```python
from build123d import *

# Parameters (mm, degrees)
SKETCH_1_W      = 60
SKETCH_1_H      = 60
EXTRUDE_1_DEPTH = 3
SKETCH_2_W      = 60
SKETCH_2_H      = 60
EXTRUDE_2_DEPTH = 35
EXTRUDE_3_DEPTH = 8


with BuildPart() as part:
    # 草图1 → 凸台-拉伸1 (new body)
    with BuildSketch(Plane(origin=(0, 0, 0), x_dir=(1, 0, 0), z_dir=(0, 1, 0))):
        Rectangle(SKETCH_1_W, SKETCH_1_H)
    extrude(amount=EXTRUDE_1_DEPTH)

    # 草图2 → 凸台-拉伸2 (add)
    with BuildSketch(Plane(origin=(0, 0, 0), x_dir=(1, 0, 0), z_dir=(0, 1, 0))):
        Polygon((-30, 32), (32, 32), (32, -32), (-32, -32), (-32, 32), align=None)
        Rectangle(SKETCH_2_W, SKETCH_2_H, mode=Mode.SUBTRACT)
    extrude(amount=EXTRUDE_2_DEPTH)

    # 草图3 → 凸台-拉伸3 (add)
    with BuildSketch(Plane.XY.offset(32)):
        with BuildLine():
            Line((-4.210680383, 19.255087703), (4.561970296, 19.255087703))
            ThreePointArc((4.561970296, 19.255087703), (6.317057998, 17.5), (4.561970296, 15.744912297))
            Line((4.561970296, 15.744912297), (-4.210680383, 15.744912297))
            ThreePointArc((-4.210680383, 15.744912297), (-5.965768086, 17.5), (-4.210680383, 19.255087703))
        make_face()
    extrude(amount=EXTRUDE_3_DEPTH)


solid = part.part
```
Geometry: final body of the model. Coordinates: model frame, mm. A direction names the side the tool comes from. Give positions to 0.01 mm unless a question says otherwise; leave off trailing zeros. Loops run counter-clockwise (first coordinate to the right, second up) from the corner with the lowest first, then second, coordinate; pieces in that order, holes last. Notation, with made-up numbers: (-35, 56.5) -> (-6, 56.5) arc R28 ccw to (-6, 92.5) -> close; hole circle Ø9 at (43.25, -37). An arc over 180 degrees is marked (long way). Use CSV: the item, a comma, the result in double quotes.
(1) Cut plane C-C (z = -12.5). Output: boundary loops of the cut face in (x, y).
From the geometry:
outline,"(-32, 0) -> (32, 0) -> (32, 35) -> (30, 35) -> (30, 3) -> (-30, 3) -> (-30, 35) -> (-32, 35) -> close"
(2) Ray query, line 1 along X through (y, z) = (32, 9); line 2 along Y through (x, z) = (-12, -12.5). Return the intervals inside material, ascending. Write a range as [from, to].
From the geometry:
line 1,"[-32, -30], [30, 32]"
line 2,"[0, 3]"
(3) Cut plane A-A (y = 12.5). Output: boundary loops of the cut face in (x, z), plus the area to 3 significant figures.
From the geometry:
outline,"(-32, -32) -> (32, -32) -> (32, 32) -> (-32, 32) -> close; hole (-30, -30) -> (30, -30) -> (30, 30) -> (-30, 30) -> close"
area,"496 mm^2"
(4) Cut plane D-D (y = 17.5). Output: boundary loops of the cut face in (x, z), plus the area to 3 significant figures.
From the geometry:
outline,"(-32, -32) -> (32, -32) -> (32, 32) -> (6.32, 32) -> (6.32, 40) -> (-5.97, 40) -> (-5.97, 32) -> (-32, 32) -> close; hole (-30, -30) -> (30, -30) -> (30, 30) -> (-30, 30) -> close"
area,"594 mm^2"
(5) First-contact query: P1, Ø4, axis at x = -8.5, y = 22.5, coming from the +Z side; P2, Ø4, axis at x = 1, z = 36, coming from the -Y side; P3, Ø2, axis at x = 18, z = -16, coming from the +Y side. Flat tips, straight axial feed; report the tip coordinate or a pass-through.
From the geometry:
P1,"z = 32"
P2,"y = 15.74"
P3,"y = 3"
(6) Pull-direction query (X, two-part tool) for faces 6 (the face through (30, 19, 0)), 7 (the face through (0, 0, 0)), 8 (the face through (-5.965, 17.461, 35.944)), 9 (the face through (-30, 19, 0)); classes: released by +X, released by -X, zero draft, split by the parting line, or undercut.
From the geometry:
face 6,"undercut"
face 7,"zero draft"
face 8,"released by -X"
face 9,"undercut"
(7) Access query for faces 1 (the face through (0, 19, 30)), 2 (the face through (6.317, 17.539, 35.944)), 3 (the face through (0, 18, 40)), 4 (the face through (0, 15.745, 36)), 5 (the face through (0, 19.255, 36)). Directions: +Z, -Z, +X, -X, +Y, -Y. A direction counts if a zero-diameter tool reaches every point of the face in a straight line with its end or side. Return the directions, or none.
From the geometry:
face 1,"+Y"
face 2,"+Z, +X"
face 3,"+Z, +X, -X, +Y, -Y"
face 4,"+Z, +X, -X, -Y"
face 5,"+Z, +X, -X, +Y"
(8) Cut plane B-B (x = -14.5). Output: boundary loops of the cut face in (y, z), plus the area to 3 significant figures.
From the geometry:
outline,"(0, -32) -> (35, -32) -> (35, -30) -> (3, -30) -> (3, 30) -> (35, 30) -> (35, 32) -> (0, 32) -> close"
area,"320 mm^2"
